For this review, use the dimensioned drawing (mm, ordinates from the lowest corner) and the shaded views. Round coordinates to 2 decimals unless told otherwise and drop trailing zeros. Write each loop counter-clockwise with the first axis right and the second up, starting at its lowest first coordinate (ties: lowest second). Pieces come first, ordered by that corner, then holes. Notation, with made-up numbers: M 89,9.5 L 108,9.5 A26 cw 108,36.5 Z; hole C -30,79 d7. An arc over 180 degrees is marked long. One line per question, with ' | ' between items. Start each with the question number.
Item 1: Add section A-A, the plane z = 0.6. State the section outline as (x, y) points, and give its area (3 significant figures).
Item 2: Add section B-B, the plane y = 45.5. State the section outline as (x, z) points.
Item 3: Add section C-C, the plane x = 75. State the section outline as (y, z) points, and give its area (3 significant figures).
Item 4: For L1, parallel to Y at x = 79.5, z = 1.55 (1 decimal); L2, parallel to X at y = 18.5, z = 0.8; L3, parallel to X at y = 52.5, z = 1.15, list the stretches that pass through material, from the lowest coordinate up.
Item 5: Add section D-D, the plane y = 17.5. State the section outline as (x, z) points.
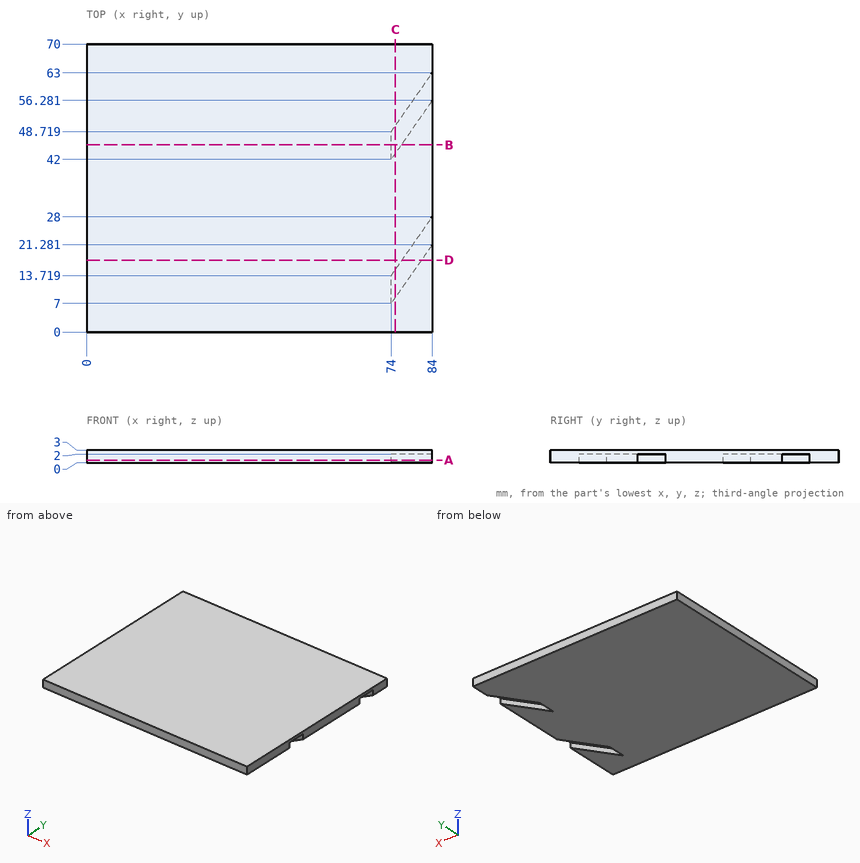
Computed values:
1) outline: M 0,0 L 84,0 L 84,21.28 L 74,7 L 74,13.72 L 84,28 L 84,56.28 L 74,42 L 74,48.72 L 84,63 L 84,70 L 0,70 Z | area: 5,750 mm^2
2) outline: M 0,0 L 74,0 L 74,2 L 76.45,2 L 76.45,0 L 84,0 L 84,3 L 0,3 Z
3) outline: M 0,0 L 8.43,0 L 8.43,2 L 15.15,2 L 15.15,0 L 43.43,0 L 43.43,2 L 50.15,2 L 50.15,0 L 70,0 L 70,3 L 0,3 Z | area: 183 mm^2
4) L1: y = 0 to 14.9, 21.6 to 49.9, 56.6 to 70 | L2: x = 0 to 77.35, 82.05 to 84 | L3: x = 0 to 76.65, 81.35 to 84
5) outline: M 0,0 L 76.65,0 L 76.65,2 L 81.35,2 L 81.35,0 L 84,0 L 84,3 L 0,3 Z
